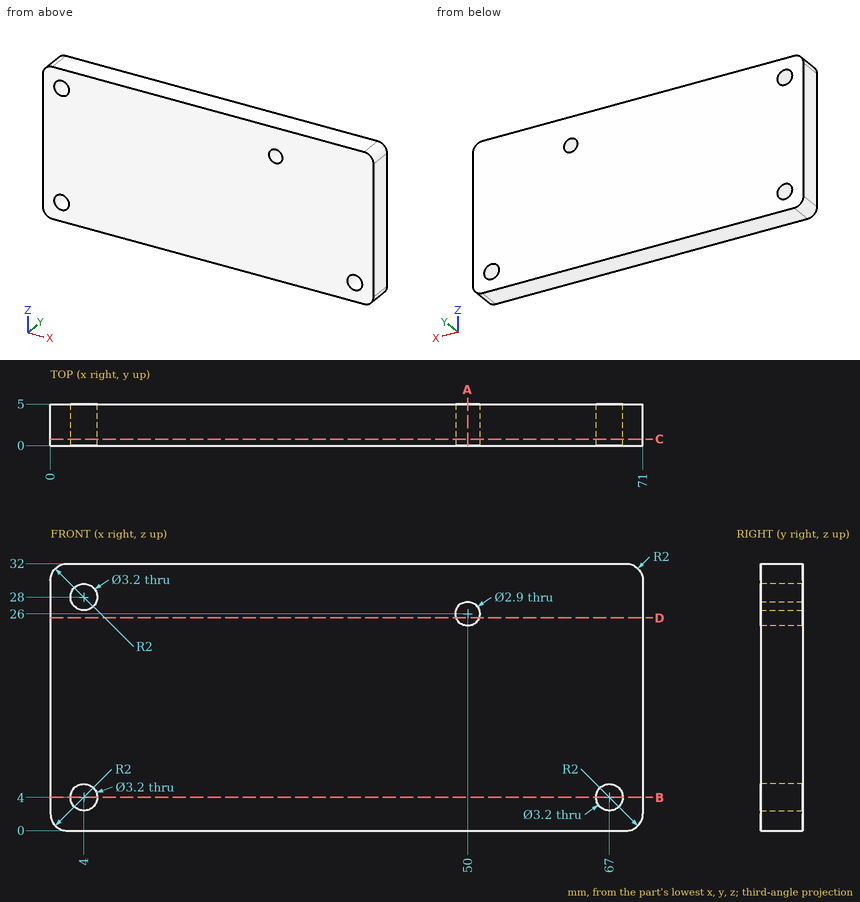
Source: three-view drawing plus pictorial views. Frame: mm from the lowest corner of the part. Coordinates: 2 decimals unless noted, no trailing zeros. Loops run counter-clockwise (first coordinate to the right, second up) from the corner with the lowest first, then second, coordinate; pieces in that order, holes last. Notation, with made-up numbers: (45, 81) - (89, 81) arc R26 cw to (89, 106) - close; hole circle Ø11 at (19.25, 73.5). An arc over 180 degrees is marked (long way). Answer in a Markdown table with one row per item. Add a question column.
Item 1: Section query A-A on x = 50. Return the cut outline in (y, z).
Item 2: Section query D-D on z = 25.5. Return the cut outline in (x, y), then the cut area to 3 significant figures.
Item 3: Section query B-B on z = 4. Return the cut outline in (x, y).
Item 4: Contact query for a flat-ended pin moving along its axis: P1, Ø1.7, axis at x = 50, z = 26, coming from the +Y side. Output: stop coordinate, or through.
Item 5: Section query C-C on y = 0.8. Return the cut outline in (x, z).
Item 6: Line query: line 1 along X through (y, z) = (3.6, 4); line 2 along X through (y, z) = (1.6, 28); line 3 along Z through (x, y) = (67, 3.65). Output: solid intervals per line, ascending. Write a range as [from, to].
Recorded:
| question | item | result |
|---|---|---|
| 1 | outline | (0, 0) - (5, 0) - (5, 24.55) - (0, 24.55) - close; (0, 27.45) - (5, 27.45) - (5, 32) - (0, 32) - close |
| 2 | outline | (0, 0) - (48.64, 0) - (48.64, 5) - (0, 5) - close; (51.36, 0) - (71, 0) - (71, 5) - (51.36, 5) - close |
| 2 | area | 341 mm^2 |
| 3 | outline | (0, 0) - (2.4, 0) - (2.4, 5) - (0, 5) - close; (5.6, 0) - (65.4, 0) - (65.4, 5) - (5.6, 5) - close; (68.6, 0) - (71, 0) - (71, 5) - (68.6, 5) - close |
| 4 | P1 | through |
| 5 | outline | (0, 2) arc R2 ccw to (2, 0) - (69, 0) arc R2 ccw to (71, 2) - (71, 30) arc R2 ccw to (69, 32) - (2, 32) arc R2 ccw to (0, 30) - close; hole circle Ø3.2 at (4, 4); hole circle Ø3.2 at (4, 28); hole circle Ø2.9 at (50, 26); hole circle Ø3.2 at (67, 4) |
| 6 | line 1 | [0, 2.4], [5.6, 65.4], [68.6, 71] |
| 6 | line 2 | [0, 2.4], [5.6, 71] |
| 6 | line 3 | [0, 2.4], [5.6, 32] |
